Autodesk Inventor part; units mm, degrees
ref_plane "Work Plane1" through (0, 0, 0) normal (0, 1, 0) x (-1, 0, 0)
ref_plane "YZ Plane" through (0, 0, 0) normal (1, 0, 0) x (0, 1, 0)
ref_plane "XY Plane" through (0, 0, 0) normal (0, 0, 1) x (1, 0, 0)
sketch "Sketch1" plane through (0, 0, 0) normal (0, 1, 0) x (-1, 0, 0)
  line L0 (0, 0) -> (5.5, 0)
  line L1 (0, 0) -> (0, -5.5)
  line L2 (0, -5.5) -> (-4.7631, -2.75)
  line L3 (-4.7631, -2.75) -> (-4.7631, 2.75)
  line L4 (-4.7631, 2.75) -> (0, 5.5)
  line L5 (0, 5.5) -> (4.7631, 2.75)
  line L6 (4.7631, 2.75) -> (4.7631, -2.75)
  line L7 (4.7631, -2.75) -> (0, -5.5)
  dimension "d0" = 5.5
  dimension "d1" = 5.5
extrude "Extrusion1" add sketch "Sketch1" along normal mid plane 4
sketch "Sketch2" plane through (0, 0, 0) normal (0, 1, 0) x (-1, 0, 0)
  circle A0 centre (0, 0) radius 4
  dimension "d4" = 8
extrude "Extrusion2" add sketch "Sketch2" along normal mid plane 20
sketch "Sketch3" plane through (0, 10, 0) normal (0, 1, 0) x (1, 0, 0)
  circle A0 centre (0, 0) radius 3
  dimension "d7" = 6
hole "Hole1" at (0, 10, 0) direction (0, -1, 0) diameter 5 depth 10 tip angle 118 counterbore diameter 6 counterbore depth 4
ref_plane "Work Plane1" through (0, 0, 0) normal (0, 1, 0) x (-1, 0, 0)
mirror "Mirror1" about plane through (0, 0, 0) normal (0, 1, 0) of "Hole1"
properties part number "Inlet Pipe Nipple"
Build history of the part. All positions in model axes, mm. A direction names the side the tool comes from. Round coordinates to 2 decimals unless told otherwise and drop trailing zeros. Write each loop counter-clockwise with the first axis right and the second up, starting at its lowest first coordinate (ties: lowest second). Pieces come first, ordered by that corner, then holes. Notation, with made-up numbers: (75.5, -25) -> (125.5, -25) arc R30 cw to (125.5, 1) -> close; hole circle Ø2 at (-25, -15.5). An arc over 180 degrees is marked (long way). Write item = value, one per line.
(1) Band-saw the part on B-B (z = 0). Give the cut face in (x, y), then the cut area to 3 significant figures.
Answer:
outline = (-4.76, -2) -> (-4, -2) -> (-4, -10) -> (-3, -10) -> (-3, -6) -> (-2.5, -6) -> (-2.5, 6) -> (-3, 6) -> (-3, 10) -> (-4, 10) -> (-4, 2) -> (-4.76, 2) -> close; (2.5, -6) -> (3, -6) -> (3, -10) -> (4, -10) -> (4, -2) -> (4.76, -2) -> (4.76, 2) -> (4, 2) -> (4, 10) -> (3, 10) -> (3, 6) -> (2.5, 6) -> close
area = 58.1 mm2
(2) Probe L1, parallel to Z at x = 0, y = 6.95; L2, parallel to X at y = 2.75, z = 0; L3, parallel to X at y = -0.5, z = 0.75. List the from-to ranges inside material, lowest first.
Answer:
L1 = -4 to -3, 3 to 4
L2 = -4 to -2.5, 2.5 to 4
L3 = -4.76 to -2.38, 2.38 to 4.76
(3) Band-saw the part on C-C (x = -1.75). Give the cut face in (y, z).
Answer:
outline = (-10, -3.6) -> (-2, -3.6) -> (-2, -4.49) -> (2, -4.49) -> (2, -3.6) -> (10, -3.6) -> (10, -2.44) -> (6, -2.44) -> (6, -1.79) -> (-6, -1.79) -> (-6, -2.44) -> (-10, -2.44) -> close; (-10, 2.44) -> (-6, 2.44) -> (-6, 1.79) -> (6, 1.79) -> (6, 2.44) -> (10, 2.44) -> (10, 3.6) -> (2, 3.6) -> (2, 4.49) -> (-2, 4.49) -> (-2, 3.6) -> (-10, 3.6) -> close
(4) Flat gauge pins, fed straight in: pin 1 (5 mm diameter, centred on x = 1, z = 2.5, fed in from -Y); pin 2 (2 mm diameter, centred on x = -2, y = -7.5, fed in from +Z); pin 3 (2 mm diameter, centred on y = 5, z = -3.5, fed in from -X); pin 4 (2 mm diameter, centred on x = 3.5, y = 5, fed in from +Z). Where does each tip first touch, or does it go through?
Answer:
pin_1 = -10
pin_2 = 3.87
pin_3 = -3.12
pin_4 = 3.12
(5) Two-plate mould, pull along Z, no slides. Class faces 4 (the face through (-4.763, 0, 0)), 5 (the face through (0.867, 5.944, 3.905)), 6 (the face through (-2, 6, -2)): pulls with the +Z half, pulls with the -Z half, needs draft (parallel to the pull), parting line crosses it, or undercut.
Answer:
face_4 = needs draft
face_5 = parting line crosses it
face_6 = undercut
(6) Band-saw the part on A-A (y = -1.5). Give the cut face in (x, z), then the cut area to 3 significant figures.
Answer:
outline = (-4.76, -2.75) -> (0, -5.5) -> (4.76, -2.75) -> (4.76, 2.75) -> (0, 5.5) -> (-4.76, 2.75) -> close; hole circle Ø5 at (0, 0)
area = 59.0 mm2
(7) Band-saw the part on D-D (x = 2.75). Give the cut face in (y, z), then the cut area to 3 significant figures.
Answer:
outline = (-10, -2.9) -> (-2, -2.9) -> (-2, -3.91) -> (2, -3.91) -> (2, -2.9) -> (10, -2.9) -> (10, -1.2) -> (6, -1.2) -> (6, 1.2) -> (10, 1.2) -> (10, 2.9) -> (2, 2.9) -> (2, 3.91) -> (-2, 3.91) -> (-2, 2.9) -> (-10, 2.9) -> (-10, 1.2) -> (-6, 1.2) -> (-6, -1.2) -> (-10, -1.2) -> close
area = 105 mm2
(8) Tool access for faces 1 (the face through (-2, -2, -4)), 2 (the face through (-2, 2, -4)), 3 (the face through (2.348, -0.028, -4.144)): list every direction of +Z, -Z, +X, -X, +Y, -Y with a clear straight run to the whole face (end or side of a thin tool).
Answer:
face_1 = -Y
face_2 = +Y
face_3 = -Z, +X, +Y, -Y
